Geometry check sheet. Reference: the model listing, model coordinates, mm. A direction names the side the tool comes from. Give positions to 0.01 mm unless a question says otherwise; leave off trailing zeros. Loops run counter-clockwise (first coordinate to the right, second up) from the corner with the lowest first, then second, coordinate; pieces in that order, holes last.
1. Material ranges on L1, parallel to Z at x = 119.5, y = -0.2; L2, parallel to Z at x = -271, y = -1.1; L3, parallel to X at y = -0.45, z = 224, recorded low to high.
2. Tool access check on faces 1 (the flat face through (-5, 0, 264)), 2 (the cylindrical face through (226.445, -0.986, -227.929)). Record the directions out of +Z, -Z, +X, -X, +Y, -Y that give a thin tool (end or side, any length) a straight path to the whole face; none if there is none.
3. Release check for a two-part mould opening along X. For faces 3 (the flat face through (-5, -2, 264)), 4 (the cylindrical face through (-226.445, -0.986, 247.929)) record: +X half, -X half, draft (parallel to the pull), parting line (faces both ways), or undercut.
4. Cross-section at B-B, the plane x = 174.5. Record the cut outline in (y, z), plus the area to 3 significant figures.
5. Cross-section at A-A, the plane z = -50.5. Record the cut outline in (x, y).
6. Cross-section at C-C, the plane y = -1.05. State how many separate pieces and enclosed holes the cut face has, plus the area to 3 significant figures.
from build123d import *

# Parameters (mm, degrees)
SKETCH1_W            = 650
SKETCH1_H            = 603.9
BASE_FLANGE1_DEPTH   = 2
M8_CLEARANCE_HOLE1_D = 9
CUT_EXTRUDE1_DEPTH   = 10
M6_CLEARANCE_HOLE1_D = 6.6
M6_CLEARANCE_HOLE2_D = 6.6
M5_CLEARANCE_HOLE1_D = 5.8
M5_CLEARANCE_HOLE2_D = 5.8
M4_CLEARANCE_HOLE1_D = 4.5
FILLET1_R            = 5


# Sheet-metal steps are written as plain solids
with BuildPart() as part:
    # Sketch1 → Base-Flange1 (new body)
    with BuildSketch(Plane(origin=(0, 0, 0), x_dir=(1, 0, 0), z_dir=(0, 1, 0))):
        Rectangle(SKETCH1_W, SKETCH1_H)
    extrude(amount=-BASE_FLANGE1_DEPTH)

    # M8 Clearance Hole1 (through all)
    with Locations(Plane(origin=(0, 0, 0), x_dir=(1, 0, 0), z_dir=(0, 1, 0))):
        with Locations((240, 286.95), (120, 286.95), (0, 286.95), (-240, 286.95), (-120, 286.95)):
            Hole(M8_CLEARANCE_HOLE1_D / 2)

    # Sketch8 → Cut-Extrude1 (cut)
    with BuildSketch(Plane(origin=(0, 0, 0), x_dir=(1, 0, 0), z_dir=(0, 1, 0))):
        with BuildLine():
            Line((205, 236.95), (-205, 236.95))
            ThreePointArc((-205, 236.95), (-226.213203436, 228.163203436), (-235, 206.95))
            Line((-235, 206.95), (-235, -226.95))
            ThreePointArc((-235, -226.95), (-226.213203436, -248.163203436), (-205, -256.95))
            Line((-205, -256.95), (205, -256.95))
            ThreePointArc((205, -256.95), (226.213203436, -248.163203436), (235, -226.95))
            Line((235, -226.95), (235, 206.95))
            ThreePointArc((235, 206.95), (226.213203436, 228.163203436), (205, 236.95))
        make_face()
    extrude(amount=-CUT_EXTRUDE1_DEPTH, mode=Mode.SUBTRACT)

    # M6 Clearance Hole1 (through all)
    with Locations(Plane(origin=(0, 0, 0), x_dir=(1, 0, 0), z_dir=(0, 1, 0))):
        with Locations((262, -164), (262, -134), (262, -104), (262, 84), (262, 114), (262, 144)):
            Hole(M6_CLEARANCE_HOLE1_D / 2)

    # M6 Clearance Hole2 (through all)
    with Locations(Plane(origin=(0, 0, 0), x_dir=(1, 0, 0), z_dir=(0, 1, 0))):
        with Locations((-271, 20), (-271, -40)):
            Hole(M6_CLEARANCE_HOLE2_D / 2)

    # M5 Clearance Hole1 (through all)
    with Locations(Plane(origin=(0, 0, 0), x_dir=(1, 0, 0), z_dir=(0, 1, 0))):
        with Locations((-316.5, 286.95), (-316.5, 196.133333333), (-316.5, 105.316666667), (-316.5, 14.5), (-316.5, -76.316666667), (-316.5, -167.133333333), (-316.5, -257.95), (-316.5, -293.45)):
            m5_clearance_hole1 = Hole(M5_CLEARANCE_HOLE1_D / 2)

    # Mirror1: M5 Clearance Hole1 across plane
    add(m5_clearance_hole1.mirror(Plane(origin=(0, 0, 0), x_dir=(0, 0, 1), z_dir=(1, 0, 0))), mode=Mode.SUBTRACT)

    # M5 Clearance Hole2 (through all)
    with Locations(Plane(origin=(0, 0, 0), x_dir=(1, 0, 0), z_dir=(0, 1, 0))):
        with Locations((-237.375, -293.45), (-158.25, -293.45), (-79.125, -293.45), (0, -293.45), (79.125, -293.45), (158.25, -293.45), (237.375, -293.45)):
            Hole(M5_CLEARANCE_HOLE2_D / 2)

    # M4 Clearance Hole1 (through all)
    with Locations(Plane(origin=(0, 0, 0), x_dir=(1, 0, 0), z_dir=(0, 1, 0))):
        with Locations((-270.6, -182.533005244), (-270.6, -204.533005244)):
            Hole(M4_CLEARANCE_HOLE1_D / 2)

    # Fillet1
    fillet1_edges = [part.edges().sort_by_distance(p)[0] for p in [
        (-325, -1, -301.95),
        (325, -1, -301.95),
        (325, -1, 301.95),
        (-325, -1, 301.95),
    ]]
    fillet(fillet1_edges, radius=FILLET1_R)


solid = part.part
Result:
1. L1: z = -301.95 to -291.42, -282.48 to -236.95, 256.95 to 301.95
1. L2: z = -301.95 to -23.3, -16.7 to 36.7, 43.3 to 180.32, 184.75 to 202.32, 206.75 to 301.95
1. L3: x = -325 to -235, 235 to 325
2. face 1: +Z, -Z, +X, -X, +Y
2. face 2: +Y, -Y
3. face 3: draft
3. face 4: undercut
4. outline: (-2, -301.95) - (0, -301.95) - (0, -236.95) - (-2, -236.95) - close; (-2, 256.95) - (0, 256.95) - (0, 301.95) - (-2, 301.95) - close
4. area: 220 mm2
5. outline: (-325, -2) - (-235, -2) - (-235, 0) - (-325, 0) - close; (235, -2) - (325, -2) - (325, 0) - (235, 0) - close
6. separate pieces: 1
6. enclosed holes: 39
6. area: 160,000 mm2
